from build123d import *

# Parameters (mm, degrees)
SKETCH1_W           = 58
SKETCH1_H           = 7
BOSS_EXTRUDE1_DEPTH = 48
CUT_EXTRUDE1_DEPTH  = 3
CUT_EXTRUDE2_DEPTH  = 3
CUT_EXTRUDE3_DEPTH  = 3
SKETCH6_R           = 1.5
BOSS_EXTRUDE2_DEPTH = 2


with BuildPart() as part:
    # Sketch1 → Boss-Extrude1 (new body)
    with BuildSketch(Plane.XY):
        with Locations((29, -3.5)):
            Rectangle(SKETCH1_W, SKETCH1_H)
    extrude(amount=BOSS_EXTRUDE1_DEPTH)

    # Sketch2 → Cut-Extrude1 (cut)
    with BuildSketch(Plane(origin=(0, 0, 0), x_dir=(1, 0, 0), z_dir=(0, 1, 0))):
        Polygon((51.5, -42.620689655), (6.5, -5.379310345), (6.5, -46.5), (51.5, -46.5), align=None)
        Polygon((6.5, -1.5), (6.5, -5.379310345), (51.5, -42.620689655), (51.5, -1.5), align=None)
    extrude(amount=-CUT_EXTRUDE1_DEPTH, mode=Mode.SUBTRACT)

    # Sketch4 → Cut-Extrude2 (cut)
    with BuildSketch(Plane.XZ.offset(7)):
        Polygon((51.5, 5.379310345), (29, 24), (6.5, 5.379310345), (6.5, 1.5), (51.5, 1.5), align=None)
        Polygon((51.5, 42.620689655), (29, 24), (51.5, 5.379310345), align=None)
        Polygon((6.5, 46.5), (6.5, 42.620689655), (29, 24), (51.5, 42.620689655), (51.5, 46.5), align=None)
        Polygon((29, 24), (6.5, 42.620689655), (6.5, 5.379310345), align=None)
    extrude(amount=-CUT_EXTRUDE2_DEPTH, mode=Mode.SUBTRACT)

    # Sketch5 → Cut-Extrude3 (cut)
    with BuildSketch(Plane(origin=(0, -3, 0), x_dir=(1, 0, 0), z_dir=(0, 1, 0))):
        with BuildLine():
            Line((51.5, -1.5), (6.5, -1.5))
            Line((6.5, -1.5), (6.5, -46.5))
            Line((6.5, -46.5), (27, -46.5))
            Line((27, -46.5), (27, -28.582575695))
            ThreePointArc((27, -28.582575695), (29, -19), (31, -28.582575695))
            Line((31, -28.582575695), (31, -46.5))
            Line((31, -46.5), (51.5, -46.5))
            Line((51.5, -46.5), (51.5, -1.5))
        make_face()
    extrude(amount=-CUT_EXTRUDE3_DEPTH, mode=Mode.SUBTRACT)

    # Sketch6 → Boss-Extrude2 (add)
    with BuildSketch(Plane(origin=(0, -3, 0), x_dir=(1, 0, 0), z_dir=(0, 1, 0))):
        with Locations(Location((29, -24, 0), (0, 0, 270))):
            Circle(SKETCH6_R)
    extrude(amount=BOSS_EXTRUDE2_DEPTH)


solid = part.part
For this review, take the finished solid that the model builds, in its own axes (mm). A direction names the side the tool comes from. Coordinates: 2 decimals unless noted, no trailing zeros. Order: outer loops, then holes, each group sorted by start corner. A loop starts at its lowest first (then second) coordinate and runs counter-clockwise, first axis right, second up. Notation, with made-up numbers: (57, 21) -> (101, 21) arc R26 ccw to (101, 43) -> close; hole circle Ø5 at (72, 56). An arc over 180 degrees is marked (long way). Return JSON: item names as keys, results as strings.
1. For line 1 (Z direction, x = 33.5, y = -2); line 2 (X direction, y = -3.25, z = 41.5); line 3 (X direction, y = -4, z = 15.5), list the stretches that pass through material, from the lowest coordinate up. Write a range as from..to.
Answer block:
{"line 1": "0..1.5, 46.5..48", "line 2": "0..6.5, 27..31, 51.5..58", "line 3": "0..6.5, 51.5..58"}
2. We need section C-C on y = -4.75. Write out the cut boundary in (x, z), and give its area (3 significant figures).
Answer block:
{"outline": "(0, 0) -> (58, 0) -> (58, 48) -> (0, 48) -> close; hole (6.5, 1.5) -> (51.5, 1.5) -> (51.5, 46.5) -> (6.5, 46.5) -> close", "area": "759 mm²"}
3. We need section D-D on z = 14.5. Write out the cut boundary in (x, y).
Answer block:
{"outline": "(0, -7) -> (6.5, -7) -> (6.5, 0) -> (0, 0) -> close; (51.5, -7) -> (58, -7) -> (58, 0) -> (51.5, 0) -> close"}
4. We need section A-A on z = 29.5. Write out the cut boundary in (x, y).
Answer block:
{"outline": "(0, -7) -> (6.5, -7) -> (6.5, 0) -> (0, 0) -> close; (27, -4) -> (31, -4) -> (31, -3) -> (27, -3) -> close; (51.5, -7) -> (58, -7) -> (58, 0) -> (51.5, 0) -> close"}
5. We need section B-B on x = 42.5. Write out the cut boundary in (y, z).
Answer block:
{"outline": "(-7, 0) -> (0, 0) -> (0, 1.5) -> (-7, 1.5) -> close; (-7, 46.5) -> (0, 46.5) -> (0, 48) -> (-7, 48) -> close"}
6. The part is to be moulded in two halves that separate along X. For faces 1 (the cylindrical face through (28.809, -3.493, 19.004)), 2 (the flat face through (29, -3, 0)), 3 (the flat face through (58, -4, 24)), 4 (the flat face through (0, -4, 24)), say which applies: +X half, -X half, draft (parallel to the pull), parting line (faces both ways), or undercut.
Answer block:
{"face 1": "undercut", "face 2": "draft", "face 3": "+X half", "face 4": "-X half"}
7. For pin 1 Ø4 at (x, y) = (25, -3) entering from -Z; pin 2 Ø11 at (x, z) = (26.5, 27) entering from +Y; pin 3 Ø5 at (x, z) = (27.5, 34) entering from -Y; pin 4 Ø12 at (x, z) = (40, 37) entering from +Y, all flat-tipped, find the tip position at first contact; note any pin that passes through.
Answer block:
{"pin 1": "z = 0", "pin 2": "y = -1", "pin 3": "y = -4", "pin 4": "through"}
8. Machinability: for faces 5 (the flat face through (29, 0, 1)), 6 (the flat face through (29, -3, 30)), 7 (the flat face through (6.5, -4, 24)), 8 (the flat face through (29, -7, 1)), 9 (the flat face through (29, -4, 30)), which of the approach directions +Z, -Z, +X, -X, +Y, -Y give a long, thin tool a straight path to every point of the face, cutting with its end or side? Answer none if there is none.
Answer block:
{"face 5": "+Z, -Z, +X, -X, +Y", "face 6": "+Y", "face 7": "+Y, -Y", "face 8": "+Z, -Z, +X, -X, -Y", "face 9": "-Y"}
